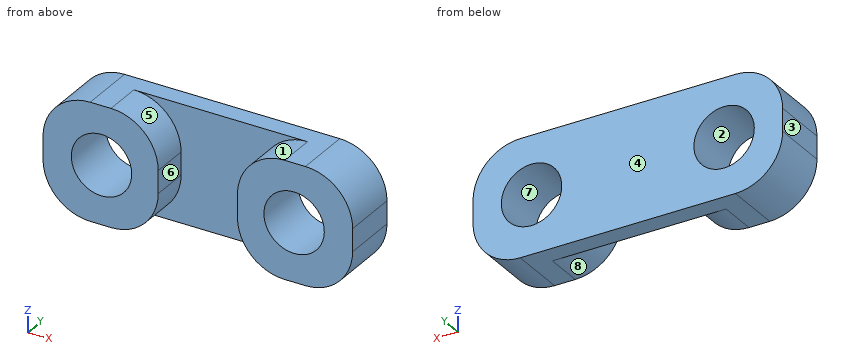
```python
from build123d import *

# Parameters (mm, degrees)
SKETCH1_W           = 16.398039
SKETCH1_H           = 6.2
SKETCH1_R           = 1.6
BOSS_EXTRUDE1_DEPTH = 3
SKETCH5_W           = 4.198039
SKETCH5_H           = 2
CUT_EXTRUDE4_DEPTH  = 11.708124054
FILLET2_R           = 2.5


with BuildPart() as part:
    # Sketch1 → Boss-Extrude1 (new body)
    with BuildSketch(Plane(origin=(0, 0, 0), x_dir=(1, 0, 0), z_dir=(0, 1, 0))):
        with Locations((0, 3.1)):
            Rectangle(SKETCH1_W, SKETCH1_H)
        with Locations(Location((-5.0990195, 3.1, 0), (0, 0, 270))):
            Circle(SKETCH1_R, mode=Mode.SUBTRACT)
        with Locations(Location((5.0990195, 3.1, 0), (0, 0, 90))):
            Circle(SKETCH1_R, mode=Mode.SUBTRACT)
    extrude(amount=BOSS_EXTRUDE1_DEPTH)

    # Sketch5 → Cut-Extrude4 (cut, through all)
    with BuildSketch(Plane.XY):
        with Locations((0, 1)):
            Rectangle(SKETCH5_W, SKETCH5_H)
    extrude(amount=-CUT_EXTRUDE4_DEPTH, mode=Mode.SUBTRACT)

    # Fillet2
    fillet2_edges = [part.edges().sort_by_distance(p)[0] for p in [
        (-2.0990195, 1, -6.2),
        (2.0990195, 1, -6.2),
        (2.0990195, 1, 0),
        (-2.0990195, 1, 0),
        (-8.1990195, 1.5, -6.2),
        (8.1990195, 1.5, -6.2),
        (8.1990195, 1.5, 0),
        (-8.1990195, 1.5, 0),
    ]]
    fillet(fillet2_edges, radius=FILLET2_R)


solid = part.part
```
Verification items for the finished model (mm, model axes). Face numbers are marked on the shaded views. A direction names the side the tool comes from. Coordinates: 2 decimals unless noted, no trailing zeros. Loops run counter-clockwise (first coordinate to the right, second up) from the corner with the lowest first, then second, coordinate; pieces in that order, holes last. Notation, with made-up numbers: (41, 11.5) - (95, 11.5) arc R18 ccw to (95, 18.5) - close; hole circle Ø5 at (47.5, 38.25). An arc over 180 degrees is marked (long way). Return JSON: item names as keys, results as strings.
1. Thickness scan on L1, parallel to X at y = 0.75, z = -3.1; L2, parallel to X at y = 2.3, z = -3.1; L3, parallel to X at y = 1.3, z = -4. Record the ranges inside material, lowest first.
Established:
{"L1": "x = -8.2 to -6.7, -3.5 to -2.1, 2.1 to 3.5, 6.7 to 8.2", "L2": "x = -8.2 to -6.7, -3.5 to 3.5, 6.7 to 8.2", "L3": "x = -8.18 to -6.42, -3.78 to -2.12, 2.12 to 3.78, 6.42 to 8.18"}
2. Section check A-A, the plane z = -3.1. Record the boundary of the cut face in (x, y).
Established:
{"outline": "(-8.2, 0) - (-6.7, 0) - (-6.7, 3) - (-8.2, 3) - close; (-3.5, 0) - (-2.1, 0) - (-2.1, 2) - (2.1, 2) - (2.1, 0) - (3.5, 0) - (3.5, 3) - (-3.5, 3) - close; (6.7, 0) - (8.2, 0) - (8.2, 3) - (6.7, 3) - close"}
3. Section check D-D, the plane z = -4. Record the boundary of the cut face in (x, y), then the cut area to 3 significant figures.
Established:
{"outline": "(-8.18, 0) - (-6.42, 0) - (-6.42, 3) - (-8.18, 3) - close; (-3.78, 0) - (-2.12, 0) - (-2.12, 2) - (2.12, 2) - (2.12, 0) - (3.78, 0) - (3.78, 3) - (-3.78, 3) - close; (6.42, 0) - (8.18, 0) - (8.18, 3) - (6.42, 3) - close", "area": "24.7 mm2"}
4. Go/stop test with flat-tipped pins: pin 1 (1.9 mm diameter, centred on x = 5.1, z = -3.1, fed in from +Y); pin 2 (3 mm diameter, centred on x = 0.5, z = -2.5, fed in from -Y); pin 3 (1 mm diameter, centred on y = 2, z = -1, fed in from +X). Record where each tip stops, or that it passes through.
Established:
{"pin 1": "passes through", "pin 2": "stops at y = 2", "pin 3": "stops at x = 7.99"}
5. Mould release check, pull along X, two halves, no side actions. Record for the marked faces 1, 2, 3 and 4: +X half, -X half, draft (parallel to the pull), parting line (faces both ways), or undercut.
Established:
{"face 1": "undercut", "face 2": "undercut", "face 3": "-X half", "face 4": "draft"}
6. Tool access check on the marked faces 5, 6, 7 and 8. Record the directions out of +Z, -Z, +X, -X, +Y, -Y that give a thin tool (end or side, any length) a straight path to the whole face; none if there is none.
Established:
{"face 5": "+Z, -Y", "face 6": "+Z, -Z, -Y", "face 7": "+Y, -Y", "face 8": "-Z, -Y"}
7. Section check B-B, the plane y = 0.95. Record the boundary of the cut face in (x, z), then the cut area to 3 significant figures.
Established:
{"outline": "(-8.2, -3.7) arc R2.5 ccw to (-5.7, -6.2) - (-4.6, -6.2) arc R2.5 ccw to (-2.1, -3.7) - (-2.1, -2.5) arc R2.5 ccw to (-4.6, 0) - (-5.7, 0) arc R2.5 ccw to (-8.2, -2.5) - close; (2.1, -3.7) arc R2.5 ccw to (4.6, -6.2) - (5.7, -6.2) arc R2.5 ccw to (8.2, -3.7) - (8.2, -2.5) arc R2.5 ccw to (5.7, 0) - (4.6, 0) arc R2.5 ccw to (2.1, -2.5) - close; hole circle Ø3.2 at (-5.1, -3.1); hole circle Ø3.2 at (5.1, -3.1)", "area": "48.8 mm2"}
8. Section check C-C, the plane x = 4. Record the boundary of the cut face in (y, z).
Established:
{"outline": "(0, -6.13) - (2, -6.13) - (2, -6.2) - (3, -6.2) - (3, -4.26) - (0, -4.26) - close; (0, -1.94) - (3, -1.94) - (3, 0) - (2, 0) - (2, -0.07) - (0, -0.07) - close"}
